Check sheet for the drawn part. Datum: minimum x, y, z corner. Units: mm. Give positions to 0.01 mm unless a question says otherwise; leave off trailing zeros. Write each loop counter-clockwise with the first axis right and the second up, starting at its lowest first coordinate (ties: lowest second). Pieces come first, ordered by that corner, then holes.
(1) Depth check by flat-ended pin: P1, Ø1.5, axis at y = 1.5, z = 1, coming from the -X side; P2, Ø0.9, axis at x = 55, y = 1, coming from the +Z side; P3, Ø1.5, axis at x = 34.5, y = 1.5, coming from the +Z side. Enter the tip coordinate at first touch or a pass-through.
(2) Cross-section at B-B (z = 39). Record the boundary of the cut face in (x, y).
(3) Thickness scan on line 1 along Z through (x, y) = (5, 2.85); line 2 along X through (y, z) = (2.7, 34.5) (1 decimal); line 3 along Z through (x, y) = (8.5, 2.15). Record the ranges inside material, lowest first.
(4) Cross-section at A-A (x = 42). Record the boundary of the cut face in (y, z).
(5) Cross-section at C-C (y = 1.1). Count the separate pieces of the cut face and the enclosed holes in it, and give its area (3 significant figures).
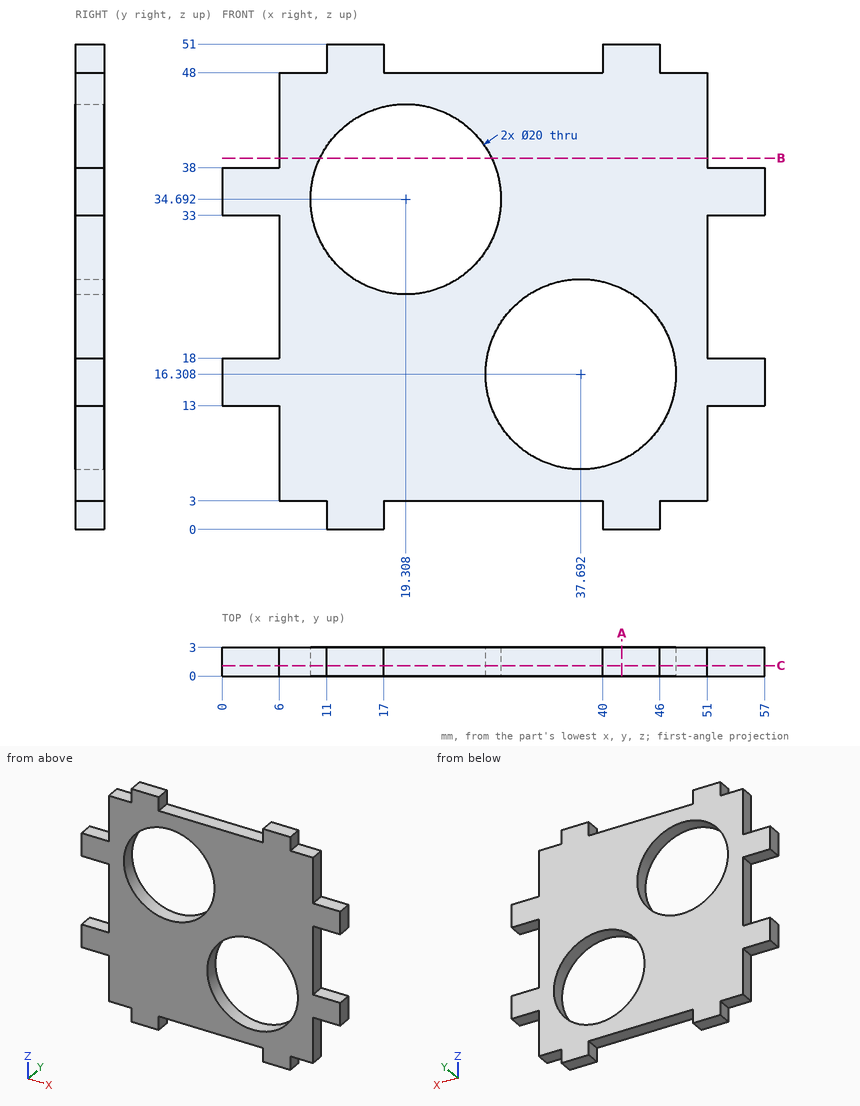
Reply:
1. P1: stops at x = 11
1. P2: stops at z = 38
1. P3: stops at z = 48
2. outline: (6, 0) - (10.28, 0) - (10.28, 3) - (6, 3) - close; (28.33, 0) - (51, 0) - (51, 3) - (28.33, 3) - close
3. line 1: z = 13 to 18, 33 to 38
3. line 2: x = 0 to 9.3, 29.3 to 57
3. line 3: z = 3 to 48
4. outline: (0, 0) - (3, 0) - (3, 7.28) - (0, 7.28) - close; (0, 25.33) - (3, 25.33) - (3, 51) - (0, 51) - close
5. separate pieces: 1
5. enclosed holes: 2
5. area: 1,590 mm2
